The listing builds one solid part. Answer for the finished solid, in the listing's coordinates (mm). A direction names the side the tool comes from. Give positions to 0.01 mm unless a question says otherwise; leave off trailing zeros. Loops run counter-clockwise (first coordinate to the right, second up) from the corner with the lowest first, then second, coordinate; pieces in that order, holes last. Notation, with made-up numbers: M 81.25,55.5 L 103.25,55.5 A37 ccw 103.25,93.5 Z; hole C 57,68 d10. An arc over 180 degrees is marked long. Return JSON: item names as keys, results as strings.
Autodesk Inventor part; units mm, degrees
ref_plane "YZ Plane" through (0, 0, 0) normal (1, 0, 0) x (0, 1, 0)
ref_plane "XZ Plane" through (0, 0, 0) normal (0, 1, 0) x (-1, 0, 0)
ref_plane "XY Plane" through (0, 0, 0) normal (0, 0, 1) x (1, 0, 0)
sketch "Sketch1" plane through (0, 0, 0) normal (1, 0, 0) x (0, 1, 0)
  arc A0 (3.4641, -2) -> (-3.4641, -2) centre (0, 0) ccw
  arc A1 (3.4641, -2) -> (5.1962, -3) centre (4.3301, -2.5) ccw
  arc A2 (-5.1962, -3) -> (-3.4641, -2) centre (-4.3301, -2.5) ccw
  line L0 (7, 16) -> (-4, 16)
  line L1 (-4, 16) -> (-4, 4.4721)
  line L2 (4.4721, 4) -> (7, 4)
  line L3 (7, 4) -> (7, 16)
  arc A3 (5.1962, -3) -> (5.8413, 1.3709) centre (0, 0) ccw
  arc A4 (-4, 4.4721) -> (-5.1962, -3) centre (0, 0) ccw
  line L4 (7, 4) -> (7, -0.8301)
  arc A5 (4.3301, -3.5) -> (7, -0.8301) centre (4.3301, -0.8301) ccw
  dimension "d0" = 8
  dimension "d4" = 2.5
  dimension "d5" = 7
  dimension "d6" = 12
  dimension "d7" = 11
  dimension "d34" = 6
  dimension "d35" = 6
extrude "Extrusion1" add sketch "Sketch1" along normal blind 38.8
fillet "Fillet1" radius 2 1 edges at (19.4, -4, 4.4721)
sketch "Sketch2" plane through (38.8, 0, 0) normal (1, 0, 0) x (0, 0, -1)
  line L0 (-16, -4) -> (-5.2915, -4)
  line L1 (-16, -4) -> (-6, -4)
  line L2 (-6, -4) -> (-6, 1.5)
  line L3 (-6, 1.5) -> (-16, 1.5)
  line L4 (-16, 1.5) -> (-16, -4)
  point P0 (0, 0)
  dimension "d11" = 10
  dimension "d12" = 5.5
extrude "Extrusion2" add sketch "Sketch2" along normal blind 3
sketch "Sketch3" plane through (0, 0, 0) normal (-1, 0, 0) x (0, 0, 1)
  point P0 (0, 0)
sketch "Sketch4" plane through (0, 0, 0) normal (-1, 0, 0) x (0, 0, 1)
  line L0 (16, -4) -> (6, -4)
  line L1 (6, -4) -> (6, 7)
  line L2 (6, 7) -> (16, 7)
  line L3 (16, 7) -> (16, -4)
  point P0 (0, 0)
  dimension "d15" = 10
  dimension "d16" = 11
extrude "Extrusion3" add sketch "Sketch4" along normal blind 4
sketch "Sketch8" plane through (-4, 0, 0) normal (-1, 0, 0) x (0, 0, 1)
  line L0 (20, 10.3) -> (30, 10.3)
  line L1 (30, 10.3) -> (30, 2.5)
  line L2 (30, 2.5) -> (20, 2.5)
  line L3 (20, 2.5) -> (20, 10.3)
  point P0 (0, 0)
  dimension "d26" = 7.8
  dimension "d27" = 10.3
  dimension "d28" = 20
  dimension "d29" = 10
extrude "Extrusion6" add sketch "Sketch8" along normal blind 6.5
sketch "Sketch9" plane through (-4, 0, 0) normal (1, 0, 0) x (0, 0, -1)
  line L0 (-30, 2.5) -> (-20, 2.5)
  line L1 (-16, 7) -> (-16, 1.5)
  line L2 (-30, 2.5) -> (-16, 2.5)
  line L3 (-16, 2.5) -> (-16, 7)
  line L4 (-16, 7) -> (-30, 7)
  line L5 (-30, 7) -> (-30, 2.5)
  point P0 (0, 0)
extrude "Extrusion7" add sketch "Sketch9" along normal blind 6
sketch "Sketch11" plane through (0, 7, 6) normal (0, 1, 0) x (1, 0, 0)
  line L0 (32.8, -8.2459) -> (12.4, -8.2459)
  line L1 (12.4, -8.2459) -> (12.4, -1.5459)
  line L2 (12.4, -1.5459) -> (32.8, -1.5459)
  line L3 (32.8, -1.5459) -> (32.8, -8.2459)
  line L4 (38.8, 6.8301) -> (38.8, -10)
  point P0 (0, 6)
  point P1 (38.8, 2)
  dimension "d47" = 20.4
  dimension "d48" = 6.7
  dimension "d67" = 6
extrude "Extrusion9" cut sketch "Sketch11" against normal blind 10
sketch "Sketch12" plane through (0, -3, 6) normal (0, 1, 0) x (1, 0, 0)
  line L0 (11.9901, -47.107) -> (11.9901, -26.707)
  line L1 (18.6901, -26.707) -> (18.6901, -47.107)
  line L2 (11.9901, -46.407) -> (18.6901, -46.407)
  line L3 (18.6901, -46.407) -> (18.6901, -43.207)
  line L4 (18.6901, -43.207) -> (11.9901, -43.207)
  line L5 (11.9901, -43.207) -> (11.9901, -46.407)
  line L6 (11.9901, -39.107) -> (18.6901, -39.107)
  line L7 (18.6901, -39.107) -> (18.6901, -35.907)
  line L8 (18.6901, -35.907) -> (11.9901, -35.907)
  line L9 (11.9901, -35.907) -> (11.9901, -39.107)
  line L10 (11.9901, -30.307) -> (18.6901, -30.307)
  line L11 (18.6901, -30.307) -> (18.6901, -27.107)
  line L12 (18.6901, -27.107) -> (11.9901, -27.107)
  line L13 (11.9901, -27.107) -> (11.9901, -30.307)
  line L14 (18.6901, -47.107) -> (11.9901, -47.107)
  line L15 (11.9901, -26.707) -> (18.6901, -26.707)
  line L16 (32.8, -8.2459) -> (12.4, -8.2459)
  line L17 (12.4, -1.5459) -> (32.8, -1.5459)
  line L18 (12.8, -8.2459) -> (16, -8.2459)
  line L19 (16, -8.2459) -> (16, -1.5459)
  line L20 (16, -1.5459) -> (12.8, -1.5459)
  line L21 (12.8, -1.5459) -> (12.8, -8.2459)
  line L22 (21.6, -8.2459) -> (24.8, -8.2459)
  line L23 (24.8, -8.2459) -> (24.8, -1.5459)
  line L24 (24.8, -1.5459) -> (21.6, -1.5459)
  line L25 (21.6, -1.5459) -> (21.6, -8.2459)
  line L26 (32.1, -8.2459) -> (28.9, -8.2459)
  line L27 (28.9, -8.2459) -> (28.9, -1.5459)
  line L28 (28.9, -1.5459) -> (32.1, -1.5459)
  line L29 (32.1, -1.5459) -> (32.1, -8.2459)
  line L30 (12.4, -8.2459) -> (12.4, -1.5459)
  point P0 (0, 6)
  point P1 (15.3401, -24.907)
  point P2 (11.9901, -44.807)
  point P3 (11.9901, -37.507)
  point P4 (11.9901, -28.707)
  point P5 (14.4, -8.2459)
  point P6 (23.2, -8.2459)
  point P7 (30.5, -8.2459)
  dimension "d51" = 7.3
  dimension "d52" = 8.8
  dimension "d53" = 3.2
  dimension "d54" = 3.2
  dimension "d55" = 3.2
  dimension "d56" = 2
  dimension "d59" = 3.2
  dimension "d60" = 3.2
  dimension "d61" = 3.2
  dimension "d62" = 8.8
  dimension "d63" = 7.3
  dimension "d64" = 2
extrude "Extrusion10" cut sketch "Sketch12" against normal blind 10 contours L16 L27 L17 L29 | L16 L25 L17 L23 | L16 L21 L17 L19
sketch "Sketch13" plane through (0, 0, 0) normal (-1, 0, 0) x (0, 0, 1)
  line L0 (-8.6099, 16.8376) -> (10, 16.8376)
  line L1 (10, -12.4202) -> (-8.6099, -12.4202)
  line L2 (-8.6099, -12.4202) -> (-8.6099, 16.8376)
  line L3 (10, 16.8376) -> (10, -12.4202)
  line L4 (16, -4) -> (16, 2.5)
  point P0 (0, 0)
  point P1 (16, 0.5)
  dimension "d70" = 6
extrude "Extrusion11" cut sketch "Sketch13" along normal mid plane 8
chamfer "Chamfer1" distance 4 angle 45 2 edges at (4, 1.5, 10) (-4, 1.5, 10)
chamfer "Chamfer2" distance 5.75 angle 45 1 edges at (2, 4.75, 16)
chamfer "Chamfer3" distance 3.3 angle 45 1 edges at (-4, 7, 25)
chamfer "Chamfer4" distance 6.5 angle 45 2 edges at (4.875, 2.5, 16) (-1, 2.5, 16)
sketch "Sketch14" plane through (38.8, 7, 16) normal (0, 1, 0) x (1, 0, 0)
  line L0 (-34.8, 10) -> (-34.8, 10.7085)
  line L1 (-34.8, 10) -> (-34.8, 7)
  line L2 (-34.8, 7) -> (-42.8, -1)
  line L3 (-42.8, 2) -> (-42.8, -4)
  line L4 (-42.8, 2) -> (-34.8, 10)
  line L5 (-42.8, 2) -> (-42.8, -1)
  line L6 (-42.8, 2) -> (-34.8, 10)
  line L7 (-42.8, -4) -> (-49.3, -4)
  point P0 (-38.8, 16)
  dimension "d85" = 3
extrude "Extrusion12" cut sketch "Sketch14" against normal blind 15
sketch "Sketch15" plane through (-10.5, 2.5, 30) normal (0, 0, 1) x (1, 0, 0)
  line L0 (0, 0) -> (12.5, 0)
  line L1 (6.5, -2.5) -> (6.5, -5.5)
  line L2 (0, 0) -> (6.5, 0)
  line L3 (6.5, 0) -> (6.5, -5.5)
  line L4 (6.5, -5.5) -> (0, -5.5)
  line L5 (0, -5.5) -> (0, 0)
  point P0 (10.5, -2.5)
extrude "Extrusion13" cut sketch "Sketch15" against normal blind 30.25
properties part number "30_Switch"
(1) Straight lines are drawn through the part: line 1 along Y through (x, z) = (14, 0); line 2 along Y through (x, z) = (14.5, 14.5); line 3 along X through (y, z) = (4.5, 25). For each, find the intervals that lie inside material, in ascending order.
Values follow:
{"line 1": "-6 to -4, 4 to 7", "line 2": "-4 to 7", "line 3": "-10.5 to 2"}
(2) The part is cut by section B-B (z = 0). Determine the outline of the cut face in (x, y).
Values follow:
{"outline": "M 4,-6 L 38.8,-6 L 38.8,-4 L 4,-4 Z; M 4,4 L 38.8,4 L 38.8,7 L 4,7 Z"}
(3) Determine the mould class of faces 1 (the cylindrical face through (21.156, -3.811, -3.355)), 2 (the flat face through (19, -3, 11)), 3 (the flat face through (4, 2, 4)), 4 (the flat face through (16, -3.5, 10.9)) for opening direction X: released by +X, released by -X, zero draft, split by the parting line, or undercut.
Values follow:
{"face 1": "zero draft", "face 2": "undercut", "face 3": "released by -X", "face 4": "undercut"}
(4) The part is cut by section C-C (x = 23). Determine the outline of the cut face in (y, z), and give its area (3 significant figures).
Values follow:
{"outline": "M -5.2,-3 A1 ccw -3.46,-2 A4 cw long 3.46,-2 A1 ccw 4.33,-3.5 A2.67 ccw 7,-0.83 L 7,7.55 L -4,7.55 L -4,5.29 A2 cw -4.5,3.97 A6 ccw Z; M -4,14.25 L 7,14.25 L 7,16 L -4,16 Z", "area": "100 mm²"}
(5) Given pin 1 (3 mm diameter, centred on x = 20.5, y = -2.5, fed in from -Z); pin 2 (2 mm diameter, centred on x = 25, z = 5.5, fed in from +Y); pin 3 (5.5 mm diameter, centred on y = 0, z = 11.5, fed in from -X), each flat-ended and moving along its own axis, determine where each tip first touches the part or whether it passes through.
Values follow:
{"pin 1": "z = -3.44", "pin 2": "y = 7", "pin 3": "x = -1.25"}
(6) A tool of negligible diameter and unlimited length cuts with its end or side. For faces 5 (the flat face through (-7, 10.3, 25)), 6 (the flat face through (2, 5, 26)), 7 (the flat face through (28.9, -3.5, 10.9)), 8 (the flat face through (12.4, 2, 11)), from which of +Z, -Z, +X, -X, +Y, -Y can it reach the whole face along a straight path? Write none if from no direction.
Values follow:
{"face 5": "+Z, -Z, +X, -X, +Y", "face 6": "+Z, +X, +Y, -Y", "face 7": "+Y, -Y", "face 8": "+Y"}
(7) The part is cut by section D-D (y = 0). Determine the outline of the cut face in (x, z), and give its area (3 significant figures).
Values follow:
{"outline": "M -4,17 L 4,9 L 4,4 L 38.8,4 L 38.8,6 L 41.8,6 L 41.8,16 L 7.75,16 L 3.75,20 L -4,20 Z; hole M 12.4,7.55 L 32.8,7.55 L 32.8,14.25 L 12.4,14.25 Z", "area": "374 mm²"}
(8) The part is cut by section A-A (z = 11). Determine the outline of the cut face in (x, y), and give its area (3 significant figures).
Values follow:
{"outline": "M 2,-4 L 12.8,-4 L 12.8,-3 L 12.4,-3 L 12.4,7 L 2,7 Z; M 16,-4 L 21.6,-4 L 21.6,-3 L 16,-3 Z; M 24.8,-4 L 28.9,-4 L 28.9,-3 L 24.8,-3 Z; M 32.1,-4 L 41.8,-4 L 41.8,1.5 L 38.8,1.5 L 38.8,7 L 32.8,7 L 32.8,-3 L 32.1,-3 Z", "area": "208 mm²"}
